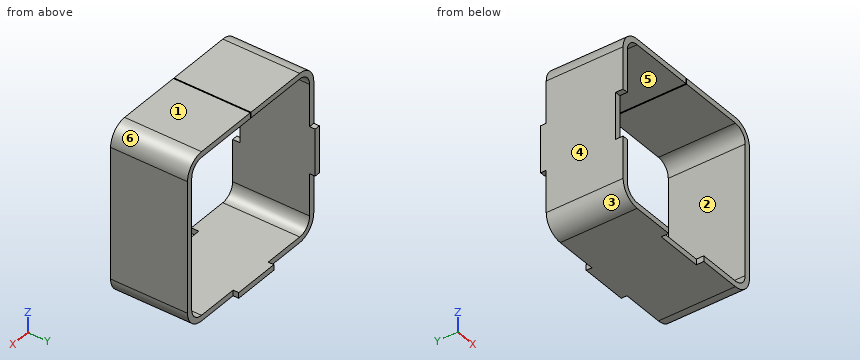
```python
from build123d import *

# Parameters (mm, degrees)
BASE_FLANGE1_DEPTH  = 41
SKETCH8_W           = 25
SKETCH8_H           = 8
CUT_EXTRUDE1_DEPTH  = 5
SKETCH9_W           = 25
SKETCH9_H           = 8
CUT_EXTRUDE2_DEPTH  = 5
SKETCH10_W          = 25
SKETCH10_H          = 6
BOSS_EXTRUDE1_DEPTH = 3
SKETCH11_W          = 25
SKETCH11_H          = 6
BOSS_EXTRUDE2_DEPTH = 3


# Read off the part's stored shape, not the designer's step: Base-Flange1
with BuildPart() as part:
    # Base-Flange1 outline → Base-Flange1 (new body)
    with BuildSketch(Plane(origin=(0, 0, 0), x_dir=(1, 0, 0), z_dir=(0, 1, 0))):
        with BuildLine():
            Line((7, -3), (41.75, -3))
            Line((41.75, -3), (41.75, 0))
            Line((41.75, 0), (7, 0))
            ThreePointArc((7, 0), (2.050252532, 2.050252532), (0, 7))
            Line((0, 7), (0, 77))
            ThreePointArc((0, 77), (2.050252532, 81.949747468), (7, 84))
            Line((7, 84), (77, 84))
            ThreePointArc((77, 84), (81.949747468, 81.949747468), (84, 77))
            Line((84, 77), (84, 7))
            ThreePointArc((84, 7), (81.949747468, 2.050252532), (77, 0))
            Line((77, 0), (42.25, 0))
            Line((42.25, 0), (42.25, -3))
            Line((42.25, -3), (77, -3))
            ThreePointArc((77, -3), (84.071067812, -0.071067812), (87, 7))
            Line((87, 7), (87, 77))
            ThreePointArc((87, 77), (84.071067812, 84.071067812), (77, 87))
            Line((77, 87), (7, 87))
            ThreePointArc((7, 87), (-0.071067812, 84.071067812), (-3, 77))
            Line((-3, 77), (-3, 7))
            ThreePointArc((-3, 7), (-0.071067812, -0.071067812), (7, -3))
        make_face()
    extrude(amount=BASE_FLANGE1_DEPTH)

    # Sketch8 → Cut-Extrude1 (cut)
    with BuildSketch(Plane(origin=(0, 0, -87), x_dir=(-1, 0, 0), z_dir=(0, 0, -1))):
        with Locations((-42, 0)):
            Rectangle(SKETCH8_W, SKETCH8_H)
    extrude(amount=-CUT_EXTRUDE1_DEPTH, mode=Mode.SUBTRACT)

    # Sketch9 → Cut-Extrude2 (cut)
    with BuildSketch(Plane.ZY.offset(3)):
        with Locations((-42, 0)):
            Rectangle(SKETCH9_W, SKETCH9_H)
    extrude(amount=-CUT_EXTRUDE2_DEPTH, mode=Mode.SUBTRACT)

    # Sketch10 → Boss-Extrude1 (add)
    with BuildSketch(Plane(origin=(0, 0, -87), x_dir=(-1, 0, 0), z_dir=(0, 0, -1))):
        with Locations((-42, 41)):
            Rectangle(SKETCH10_W, SKETCH10_H)
    extrude(amount=-BOSS_EXTRUDE1_DEPTH)

    # Sketch11 → Boss-Extrude2 (add)
    with BuildSketch(Plane.ZY.offset(3)):
        with Locations((-42, 41)):
            Rectangle(SKETCH11_W, SKETCH11_H)
    extrude(amount=-BOSS_EXTRUDE2_DEPTH)


solid = part.part
```
The listing builds one solid part. Answer for the finished solid, in the listing's coordinates (mm). Face numbers are marked on the shaded views. A direction names the side the tool comes from. Coordinates: 2 decimals unless noted, no trailing zeros. Write each loop counter-clockwise with the first axis right and the second up, starting at its lowest first coordinate (ties: lowest second). Pieces come first, ordered by that corner, then holes. Notation, with made-up numbers: (63, 38.5) - (90, 38.5) arc R21 cw to (90, 75.5) - close; hole circle Ø4 at (48, 75.25). An arc over 180 degrees is marked (long way). Return JSON: item names as keys, results as strings. Group by question number.
Q1. Which of the six approach directions +Z, -Z, +X, -X, +Y, -Y give full straight-line access (tool end or side, diameter ignored) to the marked faces 1 and 2?
Q2. Flat-ended cylindrical pins translate along their axes: pin 1 Ø2.5 at (y, z) = (42.5, -86) entering from +X; pin 2 Ø3.5 at (x, z) = (37.5, -86) entering from -Y; pin 3 Ø1.5 at (x, y) = (-2, 43) entering from +Z; pin 4 Ø22.5 at (x, z) = (70.5, -52.5) entering from +Y. Find the tip coordinate at first contact, or state that the pin passes through.
Q3. The part is cut by section B-B on x = 21. Write down the section's boundary in (y, z).
Q4. The part is cut by section A-A on z = -49. Write down the section's boundary in (x, y), and give its area (3 significant figures).
Q5. The part is cut by section C-C on y = 19. Write down the section's boundary in (x, z).
Q6. For a pull along Z with two mould halves and no side action, classify the marked faces 3, 4, 5 and 6 as +Z half, -Z half, draft (parallel to the pull), parting line (faces both ways), or undercut.
Q7. Find the intervals of material crossed by line 1 along X through (y, z) = (7, -70); line 2 along Z through (x, y) = (52, 22); line 3 along X through (y, z) = (13.5, -82.5), in increasing order. Write a range as [from, to].
Evaluation:
{
 "1": {"face 1": "+Z, +X, -X, +Y, -Y", "face 2": "+Y, -Y"},
 "2": {"pin 1": "stops at x = 54.5", "pin 2": "stops at y = 4", "pin 3": "stops at z = -29.5", "pin 4": "passes through"},
 "3": {"outline": "(0, -87) - (41, -87) - (41, -84) - (0, -84) - close; (0, 0) - (41, 0) - (41, 3) - (0, 3) - close"},
 "4": {"outline": "(-3, 4) - (0, 4) - (0, 44) - (-3, 44) - close; (84, 0) - (87, 0) - (87, 41) - (84, 41) - close", "area": "243 mm2"},
 "5": {"outline": "(-3, -77) arc R10 ccw to (7, -87) - (77, -87) arc R10 ccw to (87, -77) - (87, -7) arc R10 ccw to (77, 3) - (42.25, 3) - (42.25, 0) - (77, 0) arc R7 cw to (84, -7) - (84, -77) arc R7 cw to (77, -84) - (7, -84) arc R7 cw to (0, -77) - (0, -7) arc R7 cw to (7, 0) - (41.75, 0) - (41.75, 3) - (7, 3) arc R10 ccw to (-3, -7) - close"},
 "6": {"face 3": "-Z half", "face 4": "draft", "face 5": "undercut", "face 6": "+Z half"},
 "7": {"line 1": "x = [-3, 0], [84, 87]", "line 2": "z = [-87, -84], [0, 3]", "line 3": "x = [-1.35, 2.67], [81.33, 85.35]"}
}
